Part model, mm, in its own coordinate system. Coordinates: 2 decimals unless noted, no trailing zeros. Write each loop counter-clockwise with the first axis right and the second up, starting at its lowest first coordinate (ties: lowest second). Pieces come first, ordered by that corner, then holes. Notation, with made-up numbers: M 33,-18 L 39,-18 A6 cw 39,-7 Z; hole C 86,12 d1. An arc over 180 degrees is marked long. Use a Markdown table: item, result. Add a question column.
Q1. Slice it at B-B on x = 0. Write the cut outline in (y, z), then the cut area to 3 significant figures.
Q2. Wall check: L1, parallel to X at y = 12, z = 1.25; L2, parallel to Y at x = 8.7, z = 0.45; L3, parallel to Y at x = 0, z = -1. Give the ranges that are in metal, low to high. Write a range as from..to.
Q3. Slice it at C-C on x = -47. Write the cut outline in (y, z).
Q4. Pin check, flat tips, straight feed: pin 1 Ø3 at (y, z) = (8.5, -3.5) entering from +X; pin 2 Ø1 at (y, z) = (-23.5, 0) entering from -X; pin 3 Ø3 at (y, z) = (-11.5, 0) entering from +X. Stop position of each tip, or through.
Q5. Slice it at A-A on y = 0. Write the cut outline in (x, z), then the cut area to 4 significant figures.
Autodesk Inventor part; units mm, degrees
ref_plane "Arbeitsebene1" through (0, 0, -1) normal (0, 0, 1) x (1, 0, 0)
ref_plane "YZ Plane" through (0, 0, 0) normal (1, 0, 0) x (0, 1, 0)
ref_plane "XZ Plane" through (0, 0, 0) normal (0, 1, 0) x (-1, 0, 0)
sketch "Skizze1" plane through (0, 0, 0) normal (0, 0, 1) x (1, 0, 0)
  circle A0 centre (0, 0) radius 59.3
  circle A1 centre (0, 0) radius 52.5
  circle A2 centre (0, 0) radius 53.6 construction
  line L0 (-83.17, 0) -> (83.92, 0) construction
  line L1 (35.006, -44.9842) -> (-1.8793, -56.969)
  line L2 (-54.7615, 15.817) -> (-31.9651, 47.1935)
  line L3 (-1.8793, 56.969) -> (35.006, 44.9842)
  line L4 (-31.9651, -47.1935) -> (-54.7615, -15.817)
  arc A3 (-31.9651, -47.1935) -> (-1.8793, -56.969) centre (0, 0) ccw
  arc A4 (-54.7615, 15.817) -> (-54.7615, -15.817) centre (0, 0) ccw
  arc A5 (35.006, -44.9842) -> (35.006, 44.9842) centre (0, 0) ccw
  arc A6 (-1.8793, 56.969) -> (-31.9651, 47.1935) centre (0, 0) ccw
  circle A7 centre (0, 0) radius 46.4646
  line L5 (16.5633, -50.9766) -> (0, 0) construction
  line L6 (0, 0) -> (-43.3633, -31.5053) construction
  line L7 (0, 0) -> (16.5633, 50.9766) construction
  line L8 (0, 0) -> (-43.3633, 31.5053) construction
  point P0 (60.05, 0)
  dimension "d7" = 118.6
  dimension "d100" = 105
  dimension "d108" = 107.2
  dimension "d110" = 57
  dimension "d115" = 6.0354
  dimension "d139" = 72
  dimension "d140" = 72
  dimension "d141" = 72
  dimension "d142" = 72
extrude "Extrusion3" add sketch "Skizze1" against normal blind 5 contours L1 A3 L4 A4 L2 A6 L3 A5
extrude "Extrusion4" add sketch "Skizze1" along normal blind 1.5 contours A0 | L1 A3 L4 A4 L2 A6 L3 A5
sketch "ODroidskizze" plane through (0, 0, 1.5) normal (0, 0, 1) x (1, 0, 0)
  line L0 (0, -83.02) -> (0, 83.02) construction
  line L1 (-83.02, 0) -> (83.02, 0) construction
  line L2 (8.7, -24.5009) -> (-49.3, -24.5009) construction
  line L3 (-49.3, -24.5009) -> (-49.3, 24.4991) construction
  line L4 (-49.3, 24.4991) -> (8.7, 24.4991) construction
  line L5 (8.7, 24.4991) -> (8.7, -24.5009) construction
  line L6 (8.7, -24.5009) -> (-49.3, 24.4991) construction
  line L7 (32.7, 28.25) -> (32.7, -28.25) construction
  line L8 (32.7, -28.25) -> (-53.1757, 34.4371) construction
  line L9 (-53.1757, -34.4371) -> (32.7, 28.25) construction
  line L10 (32.7, 26.253) -> (32.7, -26.25)
  line L11 (7.2, 20.7483) -> (10.2, 20.7483)
  line L12 (12.2, 22.7483) -> (12.2, 28.25)
  line L13 (5.2, 28.25) -> (5.2, 22.7483)
  line L14 (5.2, 20.7483) -> (12.2, 28.25) construction
  line L15 (12.2, 20.7483) -> (5.2, 28.25) construction
  line L16 (7.2, -20.7517) -> (10.2, -20.7517)
  line L17 (12.2, -22.7517) -> (12.2, -28.25)
  line L18 (5.2, -28.25) -> (5.2, -22.7517)
  line L19 (5.2, -20.7517) -> (12.2, -28.25) construction
  line L20 (12.2, -20.7517) -> (5.2, -28.25) construction
  arc A0 (5.2, 22.7483) -> (7.2, 20.7483) centre (7.2, 22.7483) ccw
  arc A1 (10.2, 20.7483) -> (12.2, 22.7483) centre (10.2, 22.7483) ccw
  arc A2 (12.2, -22.7517) -> (10.2, -20.7517) centre (10.2, -22.7517) ccw
  arc A3 (7.2, -20.7517) -> (5.2, -22.7517) centre (7.2, -22.7517) ccw
  arc A4 (32.7, 26.253) -> (30.7, 28.25) centre (30.7, 26.25) ccw
  arc A5 (30.7, -28.25) -> (32.7, -26.25) centre (30.7, -26.25) ccw
  line L21 (12.2, 28.25) -> (30.7, 28.25)
  line L22 (12.2, 28.25) -> (32.7, 28.25) construction
  line L23 (30.7, -28.25) -> (12.2, -28.25)
  line L24 (32.7, -28.25) -> (12.2, -28.25) construction
  circle A6 centre (0, 0) radius 59.3
  line L25 (-42.1863, 31.25) -> (42.1863, 31.25)
  line L26 (-42.1863, -31.25) -> (42.1863, -31.25)
  line L27 (35.7, -26.25) -> (35.7, 26.25)
  line L28 (37.7, 28.25) -> (44.2514, 28.25)
  line L29 (44.2514, -28.25) -> (37.7, -28.25)
  arc A7 (37.7, 28.25) -> (35.7, 26.25) centre (37.7, 26.25) ccw
  arc A8 (35.7, -26.25) -> (37.7, -28.25) centre (37.7, -26.25) ccw
  circle A9 centre (8.7, 24.4991) radius 1.3
  circle A10 centre (8.7, -24.5009) radius 1.3
  circle A11 centre (0, 0) radius 52.5
  line L30 (-44.2514, 28.25) -> (5.2, 28.25) construction
  line L31 (-44.2514, 28.25) -> (5.2, 28.25)
  line L32 (5.2, -28.25) -> (-44.2514, -28.25)
  line L33 (5.2, -28.25) -> (-44.2514, -28.25) construction
  point P0 (0.9483, -27.9891)
  point P1 (-20.301, 0)
  point P2 (-20.301, 0)
  point P3 (-6, 0)
  point P4 (44.0485, 0)
  point P5 (-44.8148, -28.2558)
  point P6 (44.8435, -28.25)
  point P7 (44.8435, 28.25)
  point P8 (-44.8435, -28.25)
  point P9 (53, 0)
  point P10 (-53.0251, 0)
  dimension "d30" = 49
  dimension "d31" = 58
  dimension "d38" = 6
  dimension "d39" = 7
  dimension "d40" = 7
  dimension "d69" = 3
  dimension "d70" = 2
  dimension "d114" = 5.2
  dimension "d134" = 62.5
  dimension "d135" = 2.6
  dimension "d136" = 2.6
extrude "Extrusion5" add sketch "ODroidskizze" against normal blind 3.5 contours A4 L21 L12 A1 L11 A0 L13 L31 A11 L25 L28 A7 L27 A8 L29 L26 L32 L18 A3 L16 A2 L17 L23 A5 L10
ref_plane "Arbeitsebene1" through (0, 0, -1) normal (0, 0, 1) x (1, 0, 0)
sketch "Skizze8" plane through (0, 0, 1.5) normal (0, 0, 1) x (1, 0, 0)
  arc A0 (42.1863, 31.25) -> (-42.1863, 31.25) centre (0, 0) ccw construction
  arc A1 (-42.1863, -31.25) -> (42.1863, -31.25) centre (0, 0) ccw construction
  circle A2 centre (-17.9561, -49.3339) radius 2
  circle A3 centre (-17.9561, 49.3339) radius 2
  line L0 (-83.02, 0) -> (83.02, 0) construction
  line L1 (-17.9561, -49.3339) -> (0, 0) construction
  line L2 (0, 0) -> (-17.9561, 49.3339) construction
  dimension "d116" = 4
  dimension "d117" = 4
  dimension "d143" = 70
  dimension "d144" = 70
extrude "Lidar-Holder-Nose" cut sketch "Skizze8" against normal up to next
chamfer "Fase5" distance 0.5 angle 45 14 edges at (-43.3633, -31.5053, -5) (-57, 0, -5) (-17.614, -54.2102, -5) (-43.3633, 31.5053, -5) (-17.614, 54.2102, -5) (16.5633, 50.9766, -5) (57, 0, -5) (16.5633, -50.9766, -5) (-32.1969, -41.4682, 1.5) (16.0722, -49.9793, 1.5) (16.0722, 49.9793, 1.5) (-32.1969, 41.4682, 1.5) (-18.6401, 51.2132, 1.5) (-18.6401, -51.2132, 1.5)
fillet "Rundung4" radius 2 8 edges at (-44.2514, -28.25, -0.25) (44.2514, -28.25, -0.25) (44.2514, 28.25, -0.25) (-44.2514, 28.25, -0.25) (12.2, 28.25, -0.25) (5.2, 28.25, -0.25) (5.2, -28.25, -0.25) (12.2, -28.25, -0.25)
properties part number "ODroid Holder-40x" material "Kupfer, Guss"
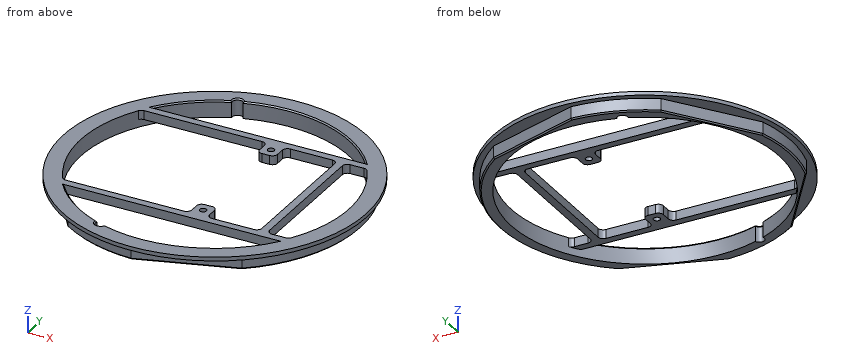
Recorded:
| question | item | result |
|---|---|---|
| 1 | outline | M -59.3,0 L -56.36,0 L -56.36,-4.5 L -55.83,-5 L -52.5,-5 L -52.5,1 L -53,1.5 L -59.3,1.5 Z; M -31.25,-2 L -28.25,-2 L -28.25,1.5 L -31.25,1.5 Z; M 28.25,-2 L 31.25,-2 L 31.25,1.5 L 28.25,1.5 Z; M 52.5,-5 L 55.83,-5 L 56.36,-4.5 L 56.36,0 L 59.3,0 L 59.3,1.5 L 53,1.5 L 52.5,1 Z |
| 1 | area | 79.5 mm² |
| 2 | L1 | -58.07..-51.11, 32.7..35.7, 51.11..58.07 |
| 2 | L2 | -58.66..-51.77, -31.25..-25.8, -23.2..-20.75, 20.75..23.2, 25.8..31.25, 51.77..58.66 |
| 2 | L3 | -56.36..-52.5, -31.25..-28.25, 28.25..31.25, 52.5..56.36 |
| 3 | outline | M -36.16,0 L -26.5,0 L -26.5,-4.5 L -25.65,-5 L -23.39,-5 L -23.39,1.5 L -36.16,1.5 Z; M 23.39,-5 L 25.65,-5 L 26.5,-4.5 L 26.5,0 L 36.16,0 L 36.16,1.5 L 23.39,1.5 Z |
| 4 | pin 1 | x = 56.57 |
| 4 | pin 2 | x = -54.66 |
| 4 | pin 3 | x = 58.45 |
| 5 | outline | M -59.3,0 L -57,0 L -57,-4.5 L -56.5,-5 L -52.5,-5 L -52.5,1.5 L -59.3,1.5 Z; M 32.7,-2 L 35.7,-2 L 35.7,1.5 L 32.7,1.5 Z; M 52.5,-5 L 56.5,-5 L 57,-4.5 L 57,0 L 59.3,0 L 59.3,1.5 L 52.5,1.5 Z |
| 5 | area | 75.65 mm² |
